Verification items for this drawing (mm, ordinates from the low corner). A direction names the side the tool comes from. Coordinates: 2 decimals unless noted, no trailing zeros. Order: outer loops, then holes, each group sorted by start corner. A loop starts at its lowest first (then second) coordinate and runs counter-clockwise, first axis right, second up. Notation, with made-up numbers: (-39.5, 50) -> (10.5, 50) arc R31 ccw to (10.5, 81) -> close; hole circle Ø10 at (88, 11.5). An arc over 180 degrees is marked (long way). Answer as CSV lines item,"result". Start each with the question number.
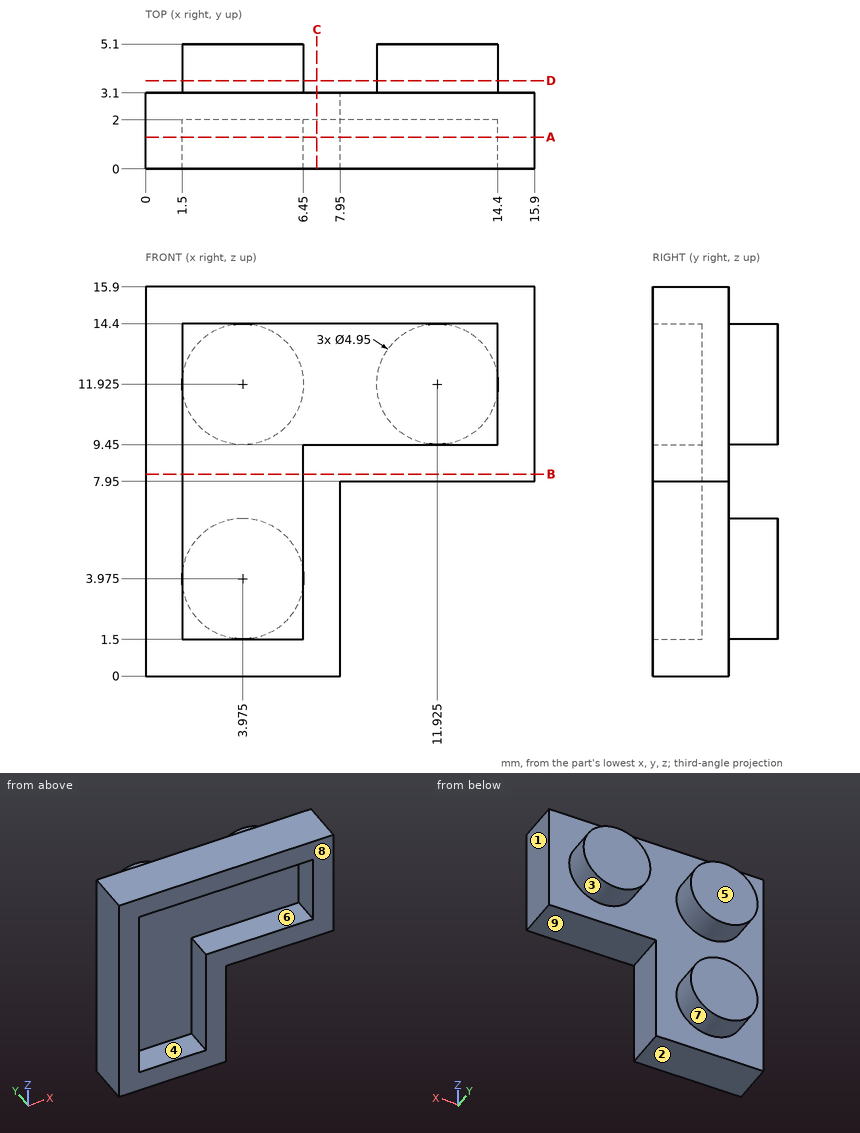
Q1. Sectioned sample at A-A, the plane y = 1.3. Record the cut outline in (x, z), then the cut area to 3 significant figures.
Q2. Sectioned sample at B-B, the plane z = 8.25. Record the cut outline in (x, y), then the cut area to 3 significant figures.
Q3. Go/stop test with flat-tipped pins: pin 1 Ø1 at (y, z) = (4.5, 14) entering from -X; pin 2 Ø1.6 at (x, y) = (13.5, 2) entering from -Z; pin 3 Ø8 at (x, z) = (8, 12.5) entering from +Y; pin 4 Ø2 at (y, z) = (1, 5) entering from +X. Record where each tip stops, or that it passes through.
Q4. Sectioned sample at C-C, the plane x = 7. Record the cut outline in (y, z).
Q5. Sectioned sample at D-D, the plane y = 3.6. Record the cut outline in (x, z) (3 decimals), then the cut area to 3 significant figures.
Q6. Thickness scan on L1, parallel to X at y = 0.45, z = 7; L2, parallel to Z at x = 5.75, y = 1.2. Record the ranges inside material, lowest first.
Q7. Release check for a two-part mould opening along X. For the marked faces 1, 2, 3 and 4 record: released by +X, released by -X, zero draft, split by the parting line, or undercut.
Q8. Access from +Z, -Z, +X, -X, +Y, -Y to the whole of each face (thin tool, end or side, straight path). Record for the marked faces 5, 6, 7, 8 and 9.
Geometry results:
1,outline,"(0, 0) -> (7.95, 0) -> (7.95, 7.95) -> (15.9, 7.95) -> (15.9, 15.9) -> (0, 15.9) -> close; hole (1.5, 1.5) -> (6.45, 1.5) -> (6.45, 9.45) -> (14.4, 9.45) -> (14.4, 14.4) -> (1.5, 14.4) -> close"
1,area,"86.4 mm^2"
2,outline,"(0, 0) -> (1.5, 0) -> (1.5, 2) -> (6.45, 2) -> (6.45, 0) -> (15.9, 0) -> (15.9, 3.1) -> (0, 3.1) -> close"
2,area,"39.4 mm^2"
3,pin 1,"stops at x = 2.07"
3,pin 2,"stops at z = 7.95"
3,pin 3,"stops at y = 5.1"
3,pin 4,"stops at x = 7.95"
4,outline,"(0, 0) -> (3.1, 0) -> (3.1, 15.9) -> (0, 15.9) -> (0, 14.4) -> (2, 14.4) -> (2, 9.45) -> (0, 9.45) -> close"
5,outline,"circle Ø4.95 at (3.975, 3.975); circle Ø4.95 at (3.975, 11.925); circle Ø4.95 at (11.925, 11.925)"
5,area,"57.7 mm^2"
6,L1,"x = 0 to 1.5, 6.45 to 7.95"
6,L2,"z = 0 to 1.5, 14.4 to 15.9"
7,face 1,"released by +X"
7,face 2,"zero draft"
7,face 3,"undercut"
7,face 4,"undercut"
8,face 5,"+Z, -Z, +X, -X, +Y"
8,face 6,"-Y"
8,face 7,"+Y"
8,face 8,"+Z, -Z, +X, -X, -Y"
8,face 9,"-Z, +X, +Y, -Y"
